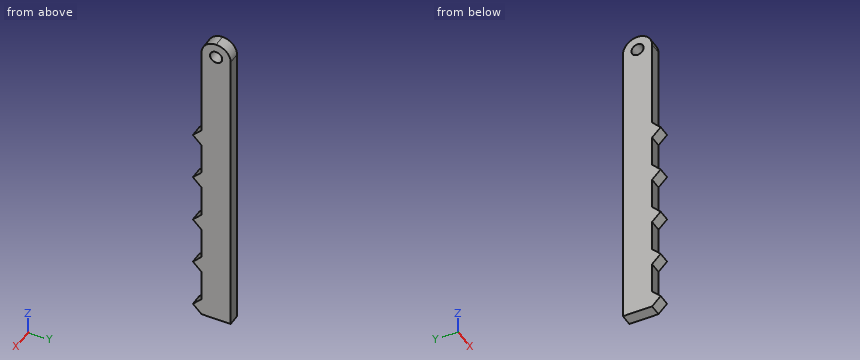
```python
from build123d import *

# Parameters (mm, degrees)
SKETCH1_W                       = 130
SKETCH1_H                       = 12
BOSS_EXTRUDE1_DEPTH             = 5
BOSS_EXTRUDE2_DEPTH             = 5
CUT_EXTRUDE1_DEPTH              = 132.020428994
F_5_0MM_DOWEL_HOLE1_D           = 5
F_5_0MM_DOWEL_HOLE1_CSINK_D     = 5.05
F_5_0MM_DOWEL_HOLE1_CSINK_ANGLE = 90


with BuildPart() as part:
    # Sketch1 → Boss-Extrude1 (new body)
    with BuildSketch(Plane(origin=(0, 0, 0), x_dir=(0, 0, -1), z_dir=(1, 0, 0))):
        with Locations((65, -6)):
            Rectangle(SKETCH1_W, SKETCH1_H)
    extrude(amount=BOSS_EXTRUDE1_DEPTH)

    # Sketch2 → Boss-Extrude2 (add)
    with BuildSketch(Plane(origin=(5, 0, 0), x_dir=(0, 0, -1), z_dir=(1, 0, 0))):
        Polygon((130, -12), (126.464466094, -15.535533906), (122.928932188, -12), align=None)
        Polygon((106.464466094, -15.535533906), (102.928932188, -12), (110, -12), align=None)
        Polygon((86.464466094, -15.535533906), (82.928932188, -12), (90, -12), align=None)
        Polygon((66.464466094, -15.535533906), (62.928932188, -12), (70, -12), align=None)
        Polygon((46.464466094, -15.535533906), (42.928932188, -12), (50, -12), align=None)
    extrude(amount=-BOSS_EXTRUDE2_DEPTH)

    # Sketch5 → Cut-Extrude1 (cut, through all)
    with BuildSketch(Plane(origin=(5, 0, 0), x_dir=(0, 0, -1), z_dir=(1, 0, 0))):
        with BuildLine():
            ThreePointArc((0, -6), (1.757359313, -1.757359313), (6, 0))
            Line((6, 0), (0, 0))
            Line((0, 0), (0, -6))
        make_face()
        with BuildLine():
            ThreePointArc((6, -12), (1.757359313, -10.242640687), (0, -6))
            Line((0, -6), (0, -12))
            Line((0, -12), (6, -12))
        make_face()
    extrude(amount=-CUT_EXTRUDE1_DEPTH, mode=Mode.SUBTRACT)

    # Ø5.0mm Dowel Hole1 (through all)
    with Locations(Plane(origin=(5, 0, 0), x_dir=(0, 0, -1), z_dir=(1, 0, 0))):
        with Locations((6, -6)):
            CounterSinkHole(F_5_0MM_DOWEL_HOLE1_D / 2, F_5_0MM_DOWEL_HOLE1_CSINK_D / 2, counter_sink_angle=F_5_0MM_DOWEL_HOLE1_CSINK_ANGLE)


solid = part.part
```
Check sheet for the modelled part. Datum: model origin and axes. Units: mm. Coordinates: 2 decimals unless noted, no trailing zeros. Write each loop counter-clockwise with the first axis right and the second up, starting at its lowest first coordinate (ties: lowest second). Pieces come first, ordered by that corner, then holes. Notation, with made-up numbers: (84.25, 88) -> (132.25, 88) arc R22 cw to (132.25, 127) -> close; hole circle Ø4 at (-8, -6). An arc over 180 degrees is marked (long way). Use a Markdown table: item, result.
1. Sectioned sample at B-B (z = -114). Enter the section's corners in (x, y), plus the area to 3 significant figures.
Reported:
| item | result |
|---|---|
| outline | (0, -12) -> (5, -12) -> (5, 0) -> (0, 0) -> close |
| area | 60.0 mm2 |
2. Sectioned sample at C-C (y = -1.5). Enter the section's corners in (x, z).
Reported:
| item | result |
|---|---|
| outline | (0, -130) -> (5, -130) -> (5, -2.03) -> (0, -2.03) -> close |
3. Sectioned sample at A-A (x = 3.85). Enter the section's corners in (y, z), plus the area to 3 significant figures.
Reported:
| item | result |
|---|---|
| outline | (-15.54, -126.46) -> (-12, -130) -> (0, -130) -> (0, -6) arc R6 ccw to (-12, -6) -> (-12, -42.93) -> (-15.54, -46.46) -> (-12, -50) -> (-12, -62.93) -> (-15.54, -66.46) -> (-12, -70) -> (-12, -82.93) -> (-15.54, -86.46) -> (-12, -90) -> (-12, -102.93) -> (-15.54, -106.46) -> (-12, -110) -> (-12, -122.93) -> close; hole circle Ø5 at (-6, -6) |
| area | 1,590 mm2 |
4. Scan lines: line 1 along Z through (x, y) = (2.75, -6); line 2 along Y through (x, z) = (2.4, -6); line 3 along Y through (x, z) = (0.6, -16). Record each from-to range of solid material in increasing order.
Reported:
| item | result |
|---|---|
| line 1 | z = -130 to -8.5, -3.5 to 0 |
| line 2 | y = -12 to -8.5, -3.5 to 0 |
| line 3 | y = -12 to 0 |
5. Go/stop test with flat-tipped pins: pin 1 Ø2.5 at (x, z) = (2, -54.5) entering from -Y; pin 2 Ø4.5 at (y, z) = (-6, -6) entering from +X; pin 3 Ø1.5 at (x, z) = (1.5, -65.5) entering from -Y. Record where each tip stops, or that it passes through.
Reported:
| item | result |
|---|---|
| pin 1 | stops at y = -12 |
| pin 2 | passes through |
| pin 3 | stops at y = -15.32 |
